from build123d import *

# Parameters (mm, degrees)
ESQUISSE1_W        = 25
ESQUISSE1_H        = 25
BOSS_EXTRU_1_DEPTH = 200
BOSS_EXTRU_2_DEPTH = 25
ESQUISSE3_R        = 25
BOSS_EXTRU_3_DEPTH = 25


with BuildPart() as part:
    # Esquisse1 → Boss.-Extru.1 (new body)
    with BuildSketch(Plane(origin=(0, 0, 0), x_dir=(1, 0, 0), z_dir=(0, 1, 0))):
        Rectangle(ESQUISSE1_W, ESQUISSE1_H)
    extrude(amount=BOSS_EXTRU_1_DEPTH)

    # Esquisse2 → Boss.-Extru.2 (add)
    with BuildSketch(Plane.XY.offset(12.5)):
        with BuildLine():
            Line((-12.5, 200), (12.5, 200))
            ThreePointArc((12.5, 200), (0, 212.5), (-12.5, 200))
        make_face()
    extrude(amount=-BOSS_EXTRU_2_DEPTH)

    # Esquisse3 → Boss.-Extru.3 (add)
    with BuildSketch(Plane.XZ):
        with Locations(Location((0, 0, 0), (0, 0, 270))):
            Circle(ESQUISSE3_R)
    extrude(amount=-BOSS_EXTRU_3_DEPTH)


solid = part.part
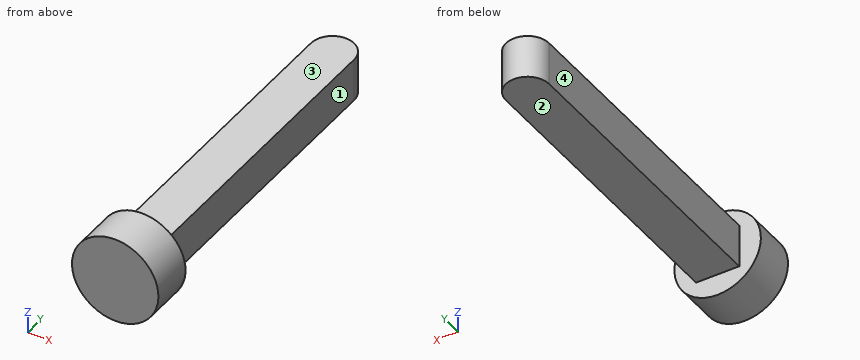
Geometry: final body of the model. Coordinates: model frame, mm. Face numbers are marked on the shaded views. A direction names the side the tool comes from. Coordinates: 2 decimals unless noted, no trailing zeros. Order: outer loops, then holes, each group sorted by start corner. A loop starts at its lowest first (then second) coordinate and runs counter-clockwise, first axis right, second up. Notation, with made-up numbers: (50, 32) - (55, 32) arc R7 ccw to (55, 40) - close; hole circle Ø4 at (-22.5, 77.5). An arc over 180 degrees is marked (long way). Use one line per item in the form item = value.
1) Pin query (flat end, axial travel): pin 1 (3 mm diameter, centred on x = 13, z = 12, fed in from +Y); pin 2 (12 mm diameter, centred on x = 7, z = 3, fed in from +Y); pin 3 (10 mm diameter, centred on x = -10, z = -10.5, fed in from +Y). Return the tip coordinate at first contact, or that it passes through.
Solutions:
pin_1 = 204.9
pin_2 = 212.46
pin_3 = 211.46
2) Set-up query: the marked faces 1, 2, 3 and 4. Return all of +Z, -Z, +X, -X, +Y, -Y with unobstructed straight access to the full face (end or side cutting, diameter ignored); none if empty.
Solutions:
face_1 = +Z, -Z, +X, +Y
face_2 = -Z, +X, -X, +Y
face_3 = +Z, +X, -X, +Y
face_4 = +Z, -Z, -X, +Y
3) Section B-B (x = 0). Return loops of the section in (y, z).
Solutions:
outline = (0, -25) - (25, -25) - (25, -12.5) - (212.5, -12.5) - (212.5, 12.5) - (25, 12.5) - (25, 25) - (0, 25) - close
4) Ray query, L1, parallel to Z at x = -3, y = 71.5; L2, parallel to Y at x = 5, z = 18. Return the intervals inside material, ascending.
Solutions:
L1 = -12.5 to 12.5
L2 = 0 to 25
5) Section D-D (x = 20). Return loops of the section in (y, z), then the cut area to 3 significant figures.
Solutions:
outline = (0, -15) - (25, -15) - (25, 15) - (0, 15) - close
area = 750 mm^2
6) Section C-C (y = 192). Return loops of the section in (x, z).
Solutions:
outline = (-12.5, -12.5) - (12.5, -12.5) - (12.5, 12.5) - (-12.5, 12.5) - close
7) Section A-A (z = 0). Return loops of the section in (x, y).
Solutions:
outline = (-25, 0) - (25, 0) - (25, 25) - (12.5, 25) - (12.5, 200) arc R12.5 ccw to (-12.5, 200) - (-12.5, 25) - (-25, 25) - close
